from build123d import *

# Parameters (mm, degrees)
EXTRUDE_1_DEPTH     = 25
CUT_EXTRUDE_1_DEPTH = 22
SKETCH_3_R          = 2.5
CUT_EXTRUDE_2_DEPTH = 72.107313267


with BuildPart() as part:
    # 草图1 → 凸台-拉伸1 (new body)
    with BuildSketch(Plane(origin=(0, 0, 0), x_dir=(1, 0, 0), z_dir=(0, 1, 0))):
        with BuildLine():
            Line((-47, 37.5), (47, 37.5))
            ThreePointArc((47, 37.5), (52.656854249, 35.156854249), (55, 29.5))
            Line((55, 29.5), (55, -29.5))
            ThreePointArc((55, -29.5), (52.656854249, -35.156854249), (47, -37.5))
            Line((47, -37.5), (-47, -37.5))
            ThreePointArc((-47, -37.5), (-52.656854249, -35.156854249), (-55, -29.5))
            Line((-55, -29.5), (-55, 29.5))
            ThreePointArc((-55, 29.5), (-52.656854249, 35.156854249), (-47, 37.5))
        make_face()
    extrude(amount=-EXTRUDE_1_DEPTH)

    # 草图2 → 切除-拉伸1 (cut)
    with BuildSketch(Plane(origin=(0, -22, 0), x_dir=(1, 0, 0), z_dir=(0, 1, 0))):
        with BuildLine():
            Line((-47, 34.5), (47, 34.5))
            ThreePointArc((47, 34.5), (50.535533906, 33.035533906), (52, 29.5))
            Line((52, 29.5), (52, -29.5))
            ThreePointArc((52, -29.5), (50.535533906, -33.035533906), (47, -34.5))
            Line((47, -34.5), (-47, -34.5))
            ThreePointArc((-47, -34.5), (-50.535533906, -33.035533906), (-52, -29.5))
            Line((-52, -29.5), (-52, 29.5))
            ThreePointArc((-52, 29.5), (-50.535533906, 33.035533906), (-47, 34.5))
        make_face()
    extrude(amount=CUT_EXTRUDE_1_DEPTH, mode=Mode.SUBTRACT)

    # 草图3 → 切除-拉伸2 (cut, through all)
    with BuildSketch(Plane(origin=(0, -25, 0), x_dir=(1, 0, 0), z_dir=(0, 1, 0))):
        with Locations(Location((-36, 18, 0), (0, 0, 90))):
            Circle(SKETCH_3_R)
        with Locations(Location((-18, 18, 0), (0, 0, 90))):
            Circle(SKETCH_3_R)
        with Locations(Location((0, 18, 0), (0, 0, 90))):
            Circle(SKETCH_3_R)
        with Locations(Location((18, 18, 0), (0, 0, 90))):
            Circle(SKETCH_3_R)
        with Locations(Location((36, 18, 0), (0, 0, 90))):
            Circle(SKETCH_3_R)
        with Locations(Location((-36, 0, 0), (0, 0, 90))):
            Circle(SKETCH_3_R)
        with Locations(Location((-18, 0, 0), (0, 0, 90))):
            Circle(SKETCH_3_R)
        with Locations(Location((0, 0, 0), (0, 0, 90))):
            Circle(SKETCH_3_R)
        with Locations(Location((18, 0, 0), (0, 0, 90))):
            Circle(SKETCH_3_R)
        with Locations(Location((36, 0, 0), (0, 0, 90))):
            Circle(SKETCH_3_R)
        with Locations(Location((-36, -18, 0), (0, 0, 90))):
            Circle(SKETCH_3_R)
        with Locations(Location((-18, -18, 0), (0, 0, 90))):
            Circle(SKETCH_3_R)
        with Locations(Location((0, -18, 0), (0, 0, 90))):
            Circle(SKETCH_3_R)
        with Locations(Location((18, -18, 0), (0, 0, 90))):
            Circle(SKETCH_3_R)
        with Locations(Location((36, -18, 0), (0, 0, 90))):
            Circle(SKETCH_3_R)
    extrude(amount=CUT_EXTRUDE_2_DEPTH, mode=Mode.SUBTRACT)


solid = part.part
Read the model definition and answer for the solid it produces. Units are mm, in the model's axes. A direction names the side the tool comes from. Round coordinates to 2 decimals unless told otherwise and drop trailing zeros. Loops run counter-clockwise (first coordinate to the right, second up) from the corner with the lowest first, then second, coordinate; pieces in that order, holes last.
Q1. This flat-tipped pin is pushed along its axis until it touches: pin 1 (1.5 mm diameter, centred on x = -10.5, z = 18, fed in from +Y). Where does it stop, or does it pass through?
Q2. Determine the mould class of faces 3 (the face through (55, -12, 0)), 4 (the face through (34.31, -23.52, -16.16)), 5 (the face through (1, -12, 37.5)) for opening direction X: released by +X, released by -X, zero draft, split by the parting line, or undercut.
Q3. Section D-D on z = -8 is taken. Write down the section's boundary in (x, y).
Q4. Consider probe 1 along X at (y, z) = (-23.95, 0); probe 2 along Z at (x, y) = (-18, -23.55); probe 3 along Z at (x, y) = (-7, -6). Determine where each line is inside the solid, lowest interval first.
Q5. Section C-C on y = -4 is taken. Write down the section's boundary in (x, z), and give its area (3 significant figures).
Q6. Section A-A on z = 18 is taken. Write down the section's boundary in (x, y), and give its area (3 significant figures).
Q7. Section B-B on x = 36 is taken. Write down the section's boundary in (y, z).
Q8. Which of the six approach directions +Z, -Z, +X, -X, +Y, -Y give full straight-line access (tool end or side, diameter ignored) to faces 1 (the face through (17.9, -23.5, -15.5)), 2 (the face through (-50.5, -11.15, 33.07))?
Output:
1. pin 1: stops at y = -22
2. face 3: released by +X
2. face 4: undercut
2. face 5: zero draft
3. outline: (-55, -25) - (55, -25) - (55, 0) - (52, 0) - (52, -22) - (-52, -22) - (-52, 0) - (-55, 0) - close
4. probe 1: x = -55 to -38.5, -33.5 to -20.5, -15.5 to -2.5, 2.5 to 15.5, 20.5 to 33.5, 38.5 to 55
4. probe 2: z = -37.5 to -20.5, -15.5 to -2.5, 2.5 to 15.5, 20.5 to 37.5
4. probe 3: z = -37.5 to -34.5, 34.5 to 37.5
5. outline: (-55, -29.5) arc R8 ccw to (-47, -37.5) - (47, -37.5) arc R8 ccw to (55, -29.5) - (55, 29.5) arc R8 ccw to (47, 37.5) - (-47, 37.5) arc R8 ccw to (-55, 29.5) - close; hole (-52, -29.5) arc R5 ccw to (-47, -34.5) - (47, -34.5) arc R5 ccw to (52, -29.5) - (52, 29.5) arc R5 ccw to (47, 34.5) - (-47, 34.5) arc R5 ccw to (-52, 29.5) - close
5. area: 1,040 mm2
6. outline: (-55, -25) - (-38.5, -25) - (-38.5, -22) - (-52, -22) - (-52, 0) - (-55, 0) - close; (-33.5, -25) - (-20.5, -25) - (-20.5, -22) - (-33.5, -22) - close; (-15.5, -25) - (-2.5, -25) - (-2.5, -22) - (-15.5, -22) - close; (2.5, -25) - (15.5, -25) - (15.5, -22) - (2.5, -22) - close; (20.5, -25) - (33.5, -25) - (33.5, -22) - (20.5, -22) - close; (38.5, -25) - (55, -25) - (55, 0) - (52, 0) - (52, -22) - (38.5, -22) - close
6. area: 387 mm2
7. outline: (-25, -37.5) - (0, -37.5) - (0, -34.5) - (-22, -34.5) - (-22, -20.5) - (-25, -20.5) - close; (-25, -15.5) - (-22, -15.5) - (-22, -2.5) - (-25, -2.5) - close; (-25, 2.5) - (-22, 2.5) - (-22, 15.5) - (-25, 15.5) - close; (-25, 20.5) - (-22, 20.5) - (-22, 34.5) - (0, 34.5) - (0, 37.5) - (-25, 37.5) - close
8. face 1: +Y, -Y
8. face 2: +Y
